Design review of the part built by this model. Coordinates are the model's own, in mm. Face numbers are marked on the shaded views. Give positions to 0.01 mm unless a question says otherwise; leave off trailing zeros. Loops run counter-clockwise (first coordinate to the right, second up) from the corner with the lowest first, then second, coordinate; pieces in that order, holes last.
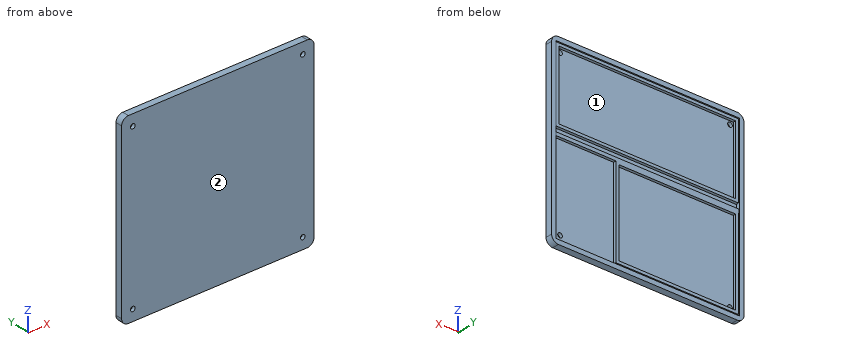
from build123d import *

# Parameters (mm, degrees)
TRAY_BODY_DEPTH              = 6
SK_POCKET_W                  = 164
SK_POCKET_H                  = 157
TRAY_POCKET_DEPTH            = 239.365265926
SK_ESP32GUIDE_W              = 163
SK_ESP32GUIDE_H              = 66.8
SK_ESP32GUIDE_W_2            = 158
SK_ESP32GUIDE_H_2            = 61.8
ESP32_HOUSING_GUIDE_DEPTH    = 2.5
SK_PI5GUIDE_W                = 109.5
SK_PI5GUIDE_H                = 81.3
SK_PI5GUIDE_W_2              = 104.5
SK_PI5GUIDE_H_2              = 76.3
PI5_CAGE_GUIDE_DEPTH         = 2.5
SK_DIVIDER_W                 = 164
SK_DIVIDER_H                 = 3
CENTER_DIVIDER_DEPTH         = 2.5
M4_MOUNTING_HOLES_DEPTH      = 239.421894968
M4_MOUNTING_HOLES_DEPTH_BACK = 239.421894968
SK_MOUNTHOLES_R              = 2.1


with BuildPart() as part:
    # Sk_Outline → Tray Body (new body)
    with BuildSketch(Plane(origin=(0, 0, 0), x_dir=(1, 0, 0), z_dir=(0, 1, 0))):
        with BuildLine():
            Line((6, 0), (166, 0))
            ThreePointArc((166, 0), (170.242640687, 1.757359313), (172, 6))
            Line((172, 6), (172, 159))
            ThreePointArc((172, 159), (170.242640687, 163.242640687), (166, 165))
            Line((166, 165), (6, 165))
            ThreePointArc((6, 165), (1.757359313, 163.242640687), (0, 159))
            Line((0, 159), (0, 6))
            ThreePointArc((0, 6), (1.757359313, 1.757359313), (6, 0))
        make_face()
    extrude(amount=TRAY_BODY_DEPTH)

    # Sk_Pocket → Tray Pocket (cut, through all)
    with BuildSketch(Plane(origin=(0, 3, 0), x_dir=(1, 0, 0), z_dir=(0, 1, 0))):
        with Locations((86, 82.5)):
            Rectangle(SK_POCKET_W, SK_POCKET_H)
    extrude(amount=TRAY_POCKET_DEPTH, mode=Mode.SUBTRACT)

    # Sk_ESP32Guide → ESP32 Housing Guide (add)
    with BuildSketch(Plane(origin=(0, 3, 0), x_dir=(1, 0, 0), z_dir=(0, 1, 0))):
        with Locations((86, 37.9)):
            Rectangle(SK_ESP32GUIDE_W, SK_ESP32GUIDE_H)
        with Locations((86, 37.9)):
            Rectangle(SK_ESP32GUIDE_W_2, SK_ESP32GUIDE_H_2, mode=Mode.SUBTRACT)
    extrude(amount=ESP32_HOUSING_GUIDE_DEPTH)

    # Sk_Pi5Guide → Pi5 Cage Guide (add)
    with BuildSketch(Plane(origin=(0, 3, 0), x_dir=(1, 0, 0), z_dir=(0, 1, 0))):
        with Locations((59.25, 119.15)):
            Rectangle(SK_PI5GUIDE_W, SK_PI5GUIDE_H)
        with Locations((59.25, 119.15)):
            Rectangle(SK_PI5GUIDE_W_2, SK_PI5GUIDE_H_2, mode=Mode.SUBTRACT)
    extrude(amount=PI5_CAGE_GUIDE_DEPTH)

    # Sk_Divider → Center Divider (add)
    with BuildSketch(Plane(origin=(0, 3, 0), x_dir=(1, 0, 0), z_dir=(0, 1, 0))):
        with Locations((86, 77.5)):
            Rectangle(SK_DIVIDER_W, SK_DIVIDER_H)
    extrude(amount=CENTER_DIVIDER_DEPTH)

    # Sk_MountHoles → M4 Mounting Holes (cut, two sides: drawn at the far end of the back side and taken through both)
    with BuildSketch(Plane(origin=(0, 0, 0), x_dir=(1, 0, 0), z_dir=(0, 1, 0)).offset(-M4_MOUNTING_HOLES_DEPTH_BACK)):
        with Locations(Location((10, 10, 0), (0, 0, 270))):
            Circle(SK_MOUNTHOLES_R)
        with Locations(Location((10, 155, 0), (0, 0, 270))):
            Circle(SK_MOUNTHOLES_R)
        with Locations(Location((162, 10, 0), (0, 0, 270))):
            Circle(SK_MOUNTHOLES_R)
        with Locations(Location((162, 155, 0), (0, 0, 270))):
            Circle(SK_MOUNTHOLES_R)
    extrude(amount=M4_MOUNTING_HOLES_DEPTH + M4_MOUNTING_HOLES_DEPTH_BACK, mode=Mode.SUBTRACT)


solid = part.part
Q1. Take a section at C-C (z = -155). Give the boundary of the cut face in (x, y).
Results:
outline: (0, 0) - (7.9, 0) - (7.9, 3) - (7, 3) - (7, 5.5) - (4.5, 5.5) - (4.5, 3) - (4, 3) - (4, 6) - (0, 6) - close; (12.1, 0) - (159.9, 0) - (159.9, 3) - (114, 3) - (114, 5.5) - (111.5, 5.5) - (111.5, 3) - (12.1, 3) - close; (164.1, 0) - (172, 0) - (172, 6) - (168, 6) - (168, 3) - (164.1, 3) - close
Q2. Draft analysis for pull direction Z (two halves, no side actions). For the marked faces 1 and 2, state which applies: pulls with the +Z half, pulls with the -Z half, needs draft (parallel to the pull), parting line crosses it, or undercut.
Results:
face 1: undercut
face 2: needs draft
Q3. Insertion check: pin 1 (6 mm diameter, centred on x = 56.5, z = -88.5, fed in from -Y). The pin has a flat end and moves straight along its axis. Give the tip position at first contact, or say it passes through.
Results:
pin 1: stops at y = 0
Q4. Wall thickness on line 1 (Z direction, x = 39, y = 3.3); line 2 (Z direction, x = 115, y = 4.5); line 3 (X direction, y = 2.15, z = -155): over which ranges is each line inside the solid? List them lowest first.
Results:
line 1: z = -165 to -161, -159.8 to -157.3, -81 to -76, -71.3 to -68.8, -7 to -4.5, -4 to 0
line 2: z = -165 to -161, -79 to -76, -71.3 to -68.8, -7 to -4.5, -4 to 0
line 3: x = 0 to 7.9, 12.1 to 159.9, 164.1 to 172
Q5. Take a section at D-D (z = -38). Give the boundary of the cut face in (x, y), plus the area to 4 significant figures.
Results:
outline: (0, 0) - (172, 0) - (172, 6) - (168, 6) - (168, 3) - (167.5, 3) - (167.5, 5.5) - (165, 5.5) - (165, 3) - (7, 3) - (7, 5.5) - (4.5, 5.5) - (4.5, 3) - (4, 3) - (4, 6) - (0, 6) - close
area: 552.5 mm2
Q6. Take a section at A-A (y = 3.95). Give the number of separate pieces and of enclosed holes in the cut face, plus the area to 3 significant figures.
Results:
separate pieces: 2
enclosed holes: 4
area: 5,090 mm2
